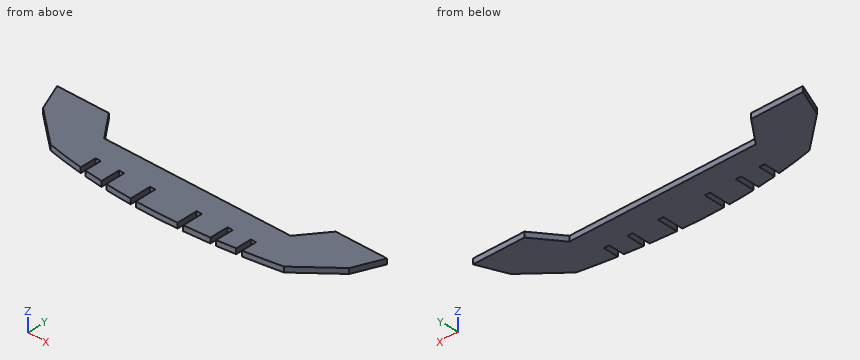
from build123d import *

# Parameters (mm, degrees)
SKETCH1_W           = 152.4
SKETCH1_H           = 38.1
BOSS_EXTRUDE1_DEPTH = 4.2926
SKETCH2_W           = 152.142509963
SKETCH2_H           = 11.43
CUT_EXTRUDE1_DEPTH  = 4.2926
SKETCH3_W           = 4.2926
SKETCH3_H           = 20.32
CUT_EXTRUDE2_DEPTH  = 4.2926


with BuildPart() as part:
    # Sketch1 → Boss-Extrude1 (new body)
    with BuildSketch(Plane.XY):
        Polygon((-83.82, 29.21), (-134.62, 29.21), (-124.968, 6.35), (-95.25, -19.05), (-76.2, -19.05), (-76.2, 19.05), align=None)
        Rectangle(SKETCH1_W, SKETCH1_H)
        with BuildLine():
            Line((-76.2, -19.05), (-95.25, -19.05))
            add(Edge.make_bspline(
                [(-95.25, -19.05), (-66.079235011, -25.514680938), (-2.12159074, -32.083739423), (61.761861898, -25.010246771), (95.25, -19.05)],
                knots=[0, 0, 0, 0, 0.467198678, 1, 1, 1, 1], degree=3))
            Line((95.25, -19.05), (76.2, -19.05))
            Line((76.2, -19.05), (-76.2, -19.05))
        make_face()
        Polygon((95.25, -19.05), (76.2, -19.05), (76.2, 19.05), (83.82, 29.21), (134.62, 29.21), (124.968, 6.35), align=None)
    extrude(amount=BOSS_EXTRUDE1_DEPTH)

    # Sketch2 → Cut-Extrude1 (cut)
    with BuildSketch(Plane.XY.offset(4.2926)):
        with Locations((-0.128745018, 13.335)):
            Rectangle(SKETCH2_W, SKETCH2_H)
    extrude(amount=-CUT_EXTRUDE1_DEPTH, mode=Mode.SUBTRACT)

    # Sketch3 → Cut-Extrude2 (cut)
    with BuildSketch(Plane.XY.offset(4.2926)):
        with Locations((-63.5, -21.59)):
            Rectangle(SKETCH3_W, SKETCH3_H)
        with Locations((-44.45, -21.59)):
            Rectangle(SKETCH3_W, SKETCH3_H)
        with Locations((-19.05, -21.59)):
            Rectangle(SKETCH3_W, SKETCH3_H)
        with Locations((44.192509963, -21.59)):
            Rectangle(SKETCH3_W, SKETCH3_H)
        with Locations((63.242509963, -21.59)):
            Rectangle(SKETCH3_W, SKETCH3_H)
        with Locations((19.05, -21.59)):
            Rectangle(SKETCH3_W, SKETCH3_H)
        Polygon((-92.3925, 29.21), (-76.2, 7.62), (-76.2, 19.05), (-83.82, 29.21), align=None)
        Polygon((75.942509963, 7.62), (92.682176292, 29.21), (83.82, 29.21), (75.942509963, 19.05), align=None)
    extrude(amount=-CUT_EXTRUDE2_DEPTH, mode=Mode.SUBTRACT)


solid = part.part
CAD build for the part. Positions are in the model's coordinates, mm. Round coordinates to 2 decimals unless told otherwise and drop trailing zeros. Order: outer loops, then holes, each group sorted by start corner. A loop starts at its lowest first (then second) coordinate and runs counter-clockwise, first axis right, second up. Notation, with made-up numbers: (68.5, 48) - (113.5, 48) arc R11 cw to (113.5, 66) - close; hole circle Ø7 at (20.5, 89). An arc over 180 degrees is marked (long way). Return JSON: item names as keys, results as strings.
(1) Cut at A-A (y = 22). Give the cut face in (x, z) (3 decimals), then the cut area to 3 significant figures.
Answer key:
{"outline": "(-131.576, 0) - (-86.985, 0) - (-86.985, 4.293) - (-131.576, 4.293) - close; (87.092, 0) - (131.576, 0) - (131.576, 4.293) - (87.092, 4.293) - close", "area": "382 mm^2"}
(2) Cut at B-B (y = -9). Give the cut face in (x, z), then the cut area to 3 significant figures.
Answer key:
{"outline": "(-107.01, 0) - (107.01, 0) - (107.01, 4.29) - (-107.01, 4.29) - close", "area": "919 mm^2"}
(3) Pin check, flat tips, straight feed: pin 1 Ø1.3 at (y, z) = (-18.5, 2.5) entering from +X; pin 2 Ø2 at (y, z) = (-17, 2) entering from +X; pin 3 Ø1.3 at (x, z) = (-45.5, 3) entering from -Y. Stop position of each tip, or through.
Answer key:
{"pin 1": "stops at x = 96.65", "pin 2": "stops at x = 98.82", "pin 3": "stops at y = -11.43"}
(4) Cut at C-C (x = 118). Give the cut face in (y, z), then the cut area to 3 significant figures.
Answer key:
{"outline": "(0.39, 0) - (29.21, 0) - (29.21, 4.29) - (0.39, 4.29) - close", "area": "124 mm^2"}
(5) Wall check: probe 1 along Y at (x, z) = (-4.5, 1.6); probe 2 along X at (y, z) = (8, 0.4) (3 decimals); probe 3 along X at (y, z) = (11.5, 2.15). Give the ranges that are in metal, low to high. Write a range as from..to.
Answer key:
{"probe 1": "y = -28.68..7.62", "probe 2": "x = -125.665..-76.485, 76.237..125.665", "probe 3": "x = -127.14..-79.11, 78.95..127.14"}
